```python
from build123d import *

# Parameters (mm, degrees)
F0_W        = 190
F0_H        = 44.5
F1_DEPTH    = 5
F2_W        = 26.885152871
F2_H        = 30.8681384815
F2_W_2      = 12.9447032342
F2_H_2      = 19
F3_DEPTH    = 5.001
F4_D        = 4.4
F5_ANGLE    = -45
F6_T1_DEPTH = 54.5
F6_T3_DEPTH = 200
F6_T5_DEPTH = 54.5


# Not quite as in the source:
# - a fillet or chamfer that OpenCascade refuses, or shapes differently, is made with other operations: its cross-section is extruded or revolved along the edge and cut away or added


with BuildPart() as f1:
    # F0 (on Top) → F1 (new body)
    with BuildSketch(Plane.XY):
        Rectangle(F0_W, F0_H)
    extrude(amount=F1_DEPTH)

    # F2 (on face) → F3 (cut, through all)
    with BuildSketch(Plane.XY.offset(5)):
        with Locations((-67.9330339405, 0)):
            Rectangle(F2_W, F2_H)
        with Locations((-29.686499387, 0.061675)):
            Rectangle(F2_W_2, F2_H_2)
        with BuildLine():
            Line((-8.9000007138, -1.3249999611), (-7.3118307668, -1.3249999611))
            ThreePointArc((-7.3118307668, -1.3249999611), (12.5999992862, 3.89e-08), (-7.3118307668, 1.3250000389))
            Line((-7.3118307668, 1.3250000389), (-8.9000007138, 1.3250000389))
            Line((-8.9000007138, 1.3250000389), (-8.9000007138, -1.3249999611))
        make_face()
        with BuildLine():
            Line((27.8544989455, -1.3249999611), (29.4426688924, -1.3249999611))
            ThreePointArc((29.4426688924, -1.3249999611), (49.3544989455, 3.89e-08), (29.4426688924, 1.3250000389))
            Line((29.4426688924, 1.3250000389), (27.8544989455, 1.3250000389))
            Line((27.8544989455, 1.3250000389), (27.8544989455, -1.3249999611))
        make_face()
        with BuildLine():
            Line((64.6044989455, -1.3293345302), (66.1926688924, -1.3293345302))
            ThreePointArc((66.1926688924, -1.3293345302), (86.1044989455, -0.0043345302), (66.1926688924, 1.3206654698))
            Line((66.1926688924, 1.3206654698), (64.6044989455, 1.3206654698))
            Line((64.6044989455, 1.3206654698), (64.6044989455, -1.3293345302))
        make_face()
    extrude(amount=-F3_DEPTH, mode=Mode.SUBTRACT)

    # F4 (through all)
    with Locations(Plane.XY.offset(5)):
        with Locations((-87.275610376, 0), (-48.590457505, 0)):
            Hole(F4_D / 2)


with BuildPart() as f1_1:
    # F5: moved
    add(f1.part.rotate(Axis((0, -22.25, 5), (-1, 0, 0)), F5_ANGLE))

    # F6: fillet of radius 2 on 4 edges, made by hand

    # F6_s2 → F6_t1 (cut)
    with BuildSketch(Plane(origin=(0, 26.3767856687, 26.3767856687), x_dir=(1, 0, 0), z_dir=(0, -0.7071067812, -0.7071067812))):
        with BuildLine():
            add(Edge.make_bspline(
                [(-95, 17.2686597873), (-95, 19.2686597873), (-93, 19.2686597873)],
                knots=[0, 0, 0, 1, 1, 1], degree=2, weights=[1, 1, 1]))
            Line((-93, 19.2686597873), (-95, 19.2686597873))
            Line((-95, 19.2686597873), (-95, 17.2686597873))
        make_face()
    extrude(amount=F6_T1_DEPTH, mode=Mode.SUBTRACT)

    # F6_s4 → F6_t3 (cut)
    with BuildSketch(Plane.YZ.offset(-100)):
        with BuildLine():
            add(Edge.make_bspline(
                [(7.8020382004, 35.0520382004), (9.2162517628, 36.4662517628), (10.6304653252, 35.0520382004)],
                knots=[0, 0, 0, 1, 1, 1], degree=2, weights=[1, 1, 1]))
            Line((10.6304653252, 35.0520382004), (9.2162517628, 36.4662517628))
            Line((9.2162517628, 36.4662517628), (7.8020382004, 35.0520382004))
        make_face()
        with BuildLine():
            add(Edge.make_bspline(
                [(-20.8357864376, 3.5857864376), (-22.25, 5), (-20.8357864376, 6.4142135624)],
                knots=[0, 0, 0, 1, 1, 1], degree=2, weights=[1, 1, 1]))
            Line((-20.8357864376, 6.4142135624), (-22.25, 5))
            Line((-22.25, 5), (-20.8357864376, 3.5857864376))
        make_face()
    extrude(amount=F6_T3_DEPTH, mode=Mode.SUBTRACT)

    # F6_s6 → F6_t5 (cut)
    with BuildSketch(Plane(origin=(0, -12.1605339059, -12.1605339059), x_dir=(1, 0, 0), z_dir=(0, 0.7071067812, 0.7071067812))):
        with BuildLine():
            add(Edge.make_bspline(
                [(95, -17.2686597873), (95, -19.2686597873), (93, -19.2686597873)],
                knots=[0, 0, 0, 1, 1, 1], degree=2, weights=[1, 1, 1]))
            Line((93, -19.2686597873), (95, -19.2686597873))
            Line((95, -19.2686597873), (95, -17.2686597873))
        make_face()
    extrude(amount=F6_T5_DEPTH, mode=Mode.SUBTRACT)


solid = f1_1.part
```
The listing builds one solid part. Answer for the finished solid, in the listing's coordinates (mm). A direction names the side the tool comes from. Round coordinates to 2 decimals unless told otherwise and drop trailing zeros. Use one line per item in the form item = value.
1. Flat-ended cylindrical pins translate along their axes: pin 1 Ø10 at (x, z) = (67, 13.5) entering from -Y; pin 2 Ø12 at (x, z) = (-44, 15.5) entering from -Y; pin 3 Ø4 at (x, z) = (-41.5, 17.5) entering from -Y; pin 4 Ø2 at (x, z) = (-67.5, 12.5) entering from -Y. Find the tip coordinate at first contact, or state that the pin passes through.
Answer key:
pin_1 = -18.75
pin_2 = -17.75
pin_3 = -11.75
pin_4 = through
2. Find the intervals of material crossed by probe 1 along X at (y, z) = (-5.5, 15); probe 2 along Z at (x, y) = (-53, 7.5); probe 3 along Y at (x, z) = (-30, 6), in increasing order. Write a range as [from, to].
Answer key:
probe_1 = [-95, -81.38], [-54.49, -36.16], [-23.21, -6.83], [12.03, 29.93], [48.78, 66.68], [85.53, 95]
probe_2 = [27.68, 34.75]
probe_3 = [-21.19, -14.18]
3. For a pull along X with two mould halves and no side action, classify faces 1 (the flat face through (-23.214, -5, 19)), 2 (the flat face through (-1.33, 4.23, 24.41)), 3 (the flat face through (95, -4, 18)) as released by +X, released by -X, zero draft, split by the parting line, or undercut.
Answer key:
face_1 = undercut
face_2 = zero draft
face_3 = released by +X
4. A tool of negligible diameter and unlimited length cuts with its end or side. For faces 4 (the flat face through (-95, -4, 18)), 5 (the flat face through (-29.78, 1.99, 25.75)), 6 (the flat face through (-36.159, -5, 19)), 7 (the flat face through (-68.12, -15.69, 8.08)), from which of +Z, -Z, +X, -X, +Y, -Y can it reach the whole face along a straight path? Write none if from no direction.
Answer key:
face_4 = +Z, -Z, -X, +Y, -Y
face_5 = -Z, -Y
face_6 = none
face_7 = +Z, +Y
